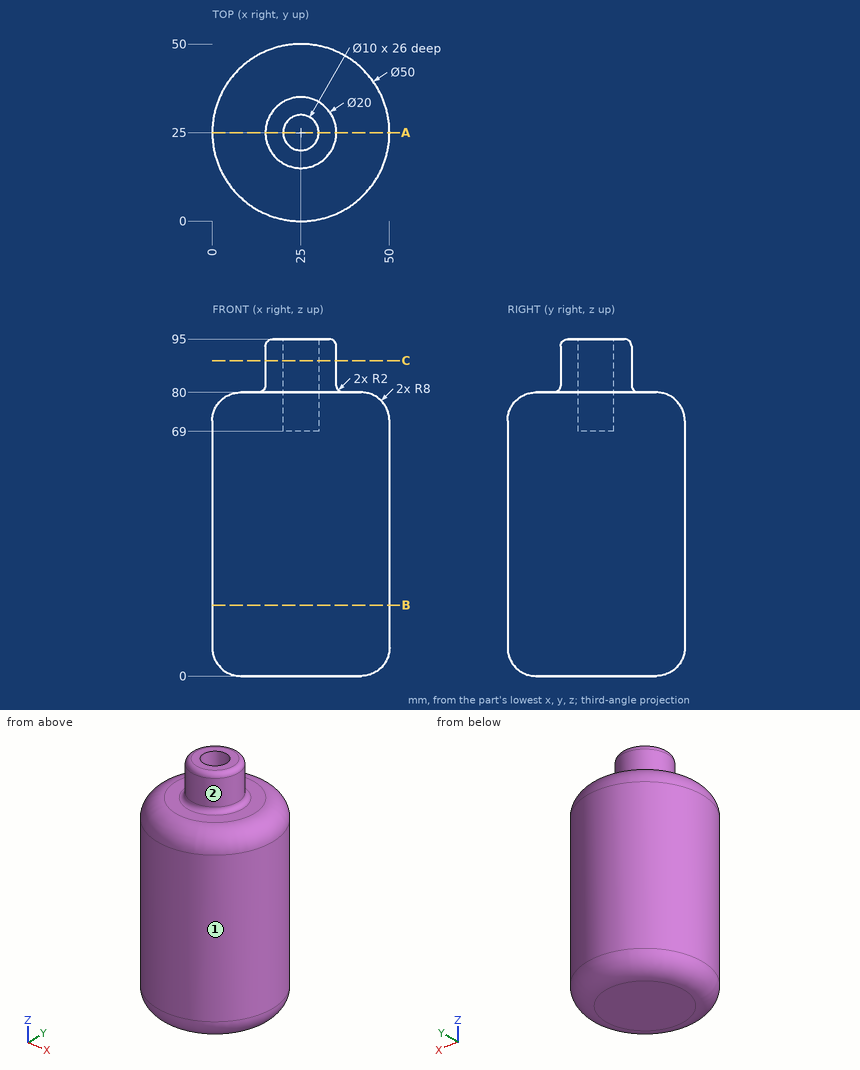
Geometry check sheet. Reference: drawing and pictorial views, mm from the part's lowest x, y, z. A direction names the side the tool comes from. Round coordinates to 2 decimals unless told otherwise and drop trailing zeros. Loops run counter-clockwise (first coordinate to the right, second up) from the corner with the lowest first, then second, coordinate; pieces in that order, holes last. Notation, with made-up numbers: M -15,-18.75 L 24,-18.75 A12 ccw 24,-6.75 Z; hole C 49.25,1.25 d3. An arc over 180 degrees is marked long. Return JSON: item names as keys, results as strings. Group by question number.
(1) Section check A-A, the plane y = 25. Enter the section's corners in (x, z), and give its area (3 significant figures).
(2) Section check C-C, the plane z = 89. Enter the section's corners in (x, y).
(3) Set-up check for the marked faces 1 and 2: record each of +Z, -Z, +X, -X, +Y, -Y from which the full face is reachable in a straight line by a thin tool's end or side.
(4) Go/stop test with flat-tipped pins: pin 1 (1 mm diameter, centred on y = 11.5, z = 79, fed in from +X); pin 2 (5 mm diameter, centred on x = 23.5, y = 25, fed in from +Z); pin 3 (4 mm diameter, centred on y = 9.5, z = 61, fed in from +X). Record where each tip stops, or that it passes through.
(5) Scan lines: line 1 along Y through (x, z) = (25, 87.5); line 2 along Z through (x, y) = (35.5, 12); line 3 along Y through (x, z) = (25, 79.25). Record each from-to range of solid material in increasing order. Write a range as [from, to].
(6) Section check B-B, the plane z = 20. Enter the section's corners in (x, y), and give its area (3 significant figures).
Data:
{
 "1": {"outline": "M 0,8 A8 ccw 8,0 L 42,0 A8 ccw 50,8 L 50,72 A8 ccw 42,80 L 37,80 A2 cw 35,82 L 35,93 A2 ccw 33,95 L 30,95 L 30,69 L 20,69 L 20,95 L 17,95 A2 ccw 15,93 L 15,82 A2 cw 13,80 L 8,80 A8 ccw 0,72 Z", "area": "3,990 mm²"},
 "2": {"outline": "C 25,25 d20; hole C 25,25 d10"},
 "3": {"face 1": "+Z, -Z", "face 2": "+Z"},
 "4": {"pin 1": "x = 42.03", "pin 2": "z = 69", "pin 3": "x = 46.04"},
 "5": {"line 1": "[15, 20], [30, 35]", "line 2": "[0, 80]", "line 3": "[4.62, 20], [30, 45.38]"},
 "6": {"outline": "C 25,25 d50", "area": "1,960 mm²"}
}
